Input: part model. Units: mm. Frame: model coordinates. Face numbers are marked on the shaded views. A direction names the side the tool comes from. Round coordinates to 2 decimals unless told otherwise and drop trailing zeros. Order: outer loops, then holes, each group sorted by start corner. A loop starts at its lowest first (then second) coordinate and runs counter-clockwise, first axis right, second up.
Item 1: Reachability of the marked faces 1 and 2 from +Z, -Z, +X, -X, +Y, -Y: full face, straight path, thin tool, end or side. Return the list, or none.
Item 2: Line query: L1, parallel to Y at x = 11, z = -5.5; L2, parallel to Z at x = 12.5, y = 5.5; L3, parallel to Y at x = -15.6, z = -25.65. Output: solid intervals per line, ascending.
Item 3: Cut plane C-C on y = 11.4. Output: boundary loops of the cut face in (x, z).
Item 4: Cut plane A-A on y = 27. Output: boundary loops of the cut face in (x, z).
Item 5: Cut plane D-D on x = -15. Output: boundary loops of the cut face in (y, z).
Item 6: Cut plane B-B on z = 13. Output: boundary loops of the cut face in (x, y).
Item 7: First-contact query: pin 1 (3.5 mm diameter, centred on x = -15.6, y = 42.6, fed in from +Z); pin 2 (12 mm diameter, centred on x = 19, z = 5.5, fed in from +Y). Flat tips, straight axial feed; report the tip coordinate or a pass-through.
```python
from build123d import *

# Parameters (mm, degrees)
SKETCH1_W           = 50
SKETCH1_H           = 50
BOSS_EXTRUDE1_DEPTH = 2
SKETCH2_W           = 50
SKETCH2_H           = 2
BOSS_EXTRUDE2_DEPTH = 52
CUT_EXTRUDE1_REACH  = 4
SKETCH3_R           = 1.6
SKETCH3_R_2         = 13.5
FILLET1_R           = 2


with BuildPart() as part:
    # Sketch1 → Boss-Extrude1 (new body)
    with BuildSketch(Plane(origin=(0, 0, 0), x_dir=(1, 0, 0), z_dir=(0, 1, 0))):
        Rectangle(SKETCH1_W, SKETCH1_H)
        with BuildLine():
            Line((-17.1, 15), (-17.1, -15))
            ThreePointArc((-17.1, -15), (-15, -17.1), (-12.9, -15))
            Line((-12.9, -15), (-12.9, 15))
            ThreePointArc((-12.9, 15), (-15, 17.1), (-17.1, 15))
        make_face(mode=Mode.SUBTRACT)
        with BuildLine():
            Line((17.1, 15), (17.1, -15))
            ThreePointArc((17.1, -15), (15, -17.1), (12.9, -15))
            Line((12.9, -15), (12.9, 15))
            ThreePointArc((12.9, 15), (15, 17.1), (17.1, 15))
        make_face(mode=Mode.SUBTRACT)
    extrude(amount=BOSS_EXTRUDE1_DEPTH)

    # Sketch2 → Boss-Extrude2 (add)
    with BuildSketch(Plane.XZ):
        with Locations((0, -26)):
            Rectangle(SKETCH2_W, SKETCH2_H)
    extrude(amount=-BOSS_EXTRUDE2_DEPTH)

    # Sketch3 → Cut-Extrude1 (cut, up to next)
    with BuildSketch(Plane.XY.offset(-25), mode=Mode.PRIVATE) as cut_extrude1_sk1:
        with Locations((-15.6, 42.6)):
            Circle(SKETCH3_R)
    cut_extrude1_tool1 = extrude(cut_extrude1_sk1.sketch, amount=-CUT_EXTRUDE1_REACH, mode=Mode.PRIVATE) & part.part
    add(cut_extrude1_tool1.solids().sort_by_distance((-15.6, 42.6, -25))[0], mode=Mode.SUBTRACT)
    # Sketch3 → Cut-Extrude1 (cut, up to next)
    with BuildSketch(Plane.XY.offset(-25), mode=Mode.PRIVATE) as cut_extrude1_sk2:
        with Locations((15.6, 42.6)):
            Circle(SKETCH3_R)
    cut_extrude1_tool2 = extrude(cut_extrude1_sk2.sketch, amount=-CUT_EXTRUDE1_REACH, mode=Mode.PRIVATE) & part.part
    add(cut_extrude1_tool2.solids().sort_by_distance((15.6, 42.6, -25))[0], mode=Mode.SUBTRACT)
    # Sketch3 → Cut-Extrude1 (cut, up to next)
    with BuildSketch(Plane.XY.offset(-25), mode=Mode.PRIVATE) as cut_extrude1_sk3:
        with Locations((15.6, 11.4)):
            Circle(SKETCH3_R)
    cut_extrude1_tool3 = extrude(cut_extrude1_sk3.sketch, amount=-CUT_EXTRUDE1_REACH, mode=Mode.PRIVATE) & part.part
    add(cut_extrude1_tool3.solids().sort_by_distance((15.6, 11.4, -25))[0], mode=Mode.SUBTRACT)
    # Sketch3 → Cut-Extrude1 (cut, up to next)
    with BuildSketch(Plane.XY.offset(-25), mode=Mode.PRIVATE) as cut_extrude1_sk4:
        with Locations((-15.6, 11.4)):
            Circle(SKETCH3_R)
    cut_extrude1_tool4 = extrude(cut_extrude1_sk4.sketch, amount=-CUT_EXTRUDE1_REACH, mode=Mode.PRIVATE) & part.part
    add(cut_extrude1_tool4.solids().sort_by_distance((-15.6, 11.4, -25))[0], mode=Mode.SUBTRACT)
    # Sketch3 → Cut-Extrude1 (cut, up to next)
    with BuildSketch(Plane.XY.offset(-25), mode=Mode.PRIVATE) as cut_extrude1_sk5:
        with Locations((0, 27)):
            Circle(SKETCH3_R_2)
    cut_extrude1_tool5 = extrude(cut_extrude1_sk5.sketch, amount=-CUT_EXTRUDE1_REACH, mode=Mode.PRIVATE) & part.part
    add(cut_extrude1_tool5.solids().sort_by_distance((0, 27, -25))[0], mode=Mode.SUBTRACT)

    # Fillet1
    fillet1_edges = [part.edges().sort_by_distance(p)[0] for p in [
        (0, 0, -27),
    ]]
    fillet(fillet1_edges, radius=FILLET1_R)


solid = part.part
```
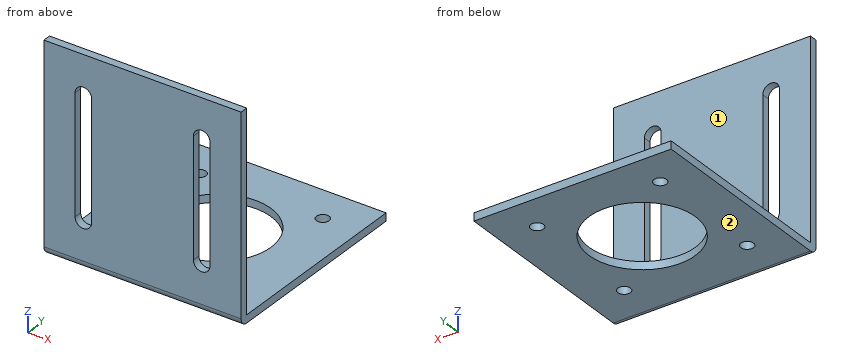
From the geometry:
1. face 1: +Z, +X, -X, +Y
1. face 2: -Z, +X, -X, +Y, -Y
2. L1: y = 0 to 2
2. L2: z = -27 to -25
2. L3: y = 0.11 to 9.8, 13 to 41, 44.2 to 52
3. outline: (-25, -27) - (-17.2, -27) - (-17.2, -25) - (-25, -25) - close; (-14, -27) - (14, -27) - (14, -25) - (-14, -25) - close; (17.2, -27) - (25, -27) - (25, -25) - (17.2, -25) - close
4. outline: (-25, -27) - (-13.5, -27) - (-13.5, -25) - (-25, -25) - close; (13.5, -27) - (25, -27) - (25, -25) - (13.5, -25) - close
5. outline: (0, -25) arc R2 ccw to (2, -27) - (9.92, -27) - (9.92, -25) - (2, -25) - (2, -17.1) - (0, -17.1) - close; (0, 17.1) - (2, 17.1) - (2, 25) - (0, 25) - close; (12.88, -27) - (41.12, -27) - (41.12, -25) - (12.88, -25) - close; (44.08, -27) - (52, -27) - (52, -25) - (44.08, -25) - close
6. outline: (-25, 0) - (-17.1, 0) - (-17.1, 2) - (-25, 2) - close; (-12.9, 0) - (12.9, 0) - (12.9, 2) - (-12.9, 2) - close; (17.1, 0) - (25, 0) - (25, 2) - (17.1, 2) - close
7. pin 1: stops at z = -25
7. pin 2: stops at y = 2
